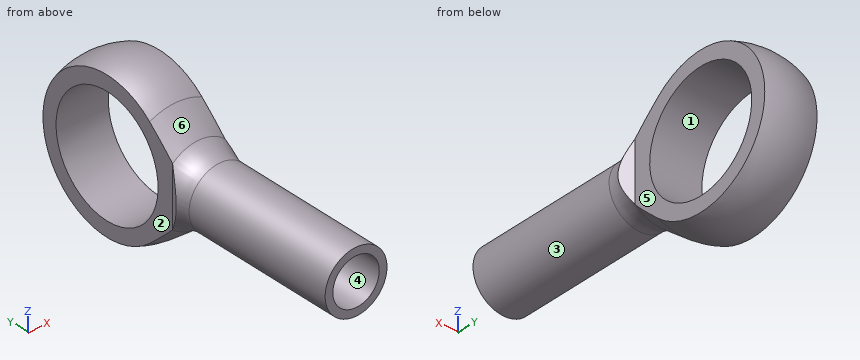
from build123d import *

# Parameters (mm, degrees)
CUT_EXTRUDE4_DEPTH      = 46.034307992
CUT_EXTRUDE4_DEPTH_BACK = 46.034307992
SKETCH3_R               = 7.5
CUT_EXTRUDE5_DEPTH      = 24
SKETCH5_R               = 3
CUT_EXTRUDE6_DEPTH      = 12.7


with BuildPart() as part:
    # Sketch1 → Revolve2 (revolve)
    with BuildSketch(Plane.XY, mode=Mode.PRIVATE) as revolve2_sk:
        with BuildLine():
            Line((0, 0), (0, 42.756156239))
            ThreePointArc((0, 42.756156239), (-9.01476789, 37.08443071), (-7.803677944, 26.502948219))
            Line((-7.803677944, 26.502948219), (-5.098161028, 23.12660401))
            ThreePointArc((-5.098161028, 23.12660401), (-4.282522133, 21.656925638), (-4, 20))
            Line((-4, 20), (-4, 0))
            Line((-4, 0), (0, 0))
        make_face()
    revolve(revolve2_sk.sketch.rotate(Axis((0, 0, 0), (0, 1, 0)), 270), axis=Axis((0, 0, 0), (0, 1, 0)))

    # Sketch2 → Cut-Extrude4 (cut, two sides: drawn at the far end of the back side and taken through both)
    with BuildSketch(Plane.XY.offset(-CUT_EXTRUDE4_DEPTH_BACK)):
        Polygon((-3.375, 42.756156239), (-20, 42.756156239), (-20, -5.668740666), (-3.375, 23.12660401), align=None)
        Polygon((20, 42.756156239), (3.375, 42.756156239), (3.375, 23.12660401), (20, -5.668740666), align=None)
    extrude(amount=CUT_EXTRUDE4_DEPTH + CUT_EXTRUDE4_DEPTH_BACK, mode=Mode.SUBTRACT)

    # Sketch3 → Cut-Extrude5 (cut)
    with BuildSketch(Plane(origin=(3.375, 0, 0), x_dir=(0, 0, -1), z_dir=(1, 0, 0))):
        with Locations((0, 32.756156239)):
            Circle(SKETCH3_R)
    extrude(amount=-CUT_EXTRUDE5_DEPTH, mode=Mode.SUBTRACT)

    # Sketch5 → Cut-Extrude6 (cut)
    with BuildSketch(Plane.XZ):
        with Locations(Location((0, 0, 0), (0, 0, 270))):
            Circle(SKETCH5_R)
    extrude(amount=-CUT_EXTRUDE6_DEPTH, mode=Mode.SUBTRACT)


solid = part.part
Design review of the part built by this model. Coordinates are the model's own, in mm. Face numbers are marked on the shaded views. A direction names the side the tool comes from. Coordinates: 2 decimals unless noted, no trailing zeros. Write each loop counter-clockwise with the first axis right and the second up, starting at its lowest first coordinate (ties: lowest second). Pieces come first, ordered by that corner, then holes. Notation, with made-up numbers: (-12.75, -30) - (-2.75, -30) arc R20 ccw to (-2.75, -3) - close; hole circle Ø11 at (-26, -19.5). An arc over 180 degrees is marked (long way). One line per item, written item: value.
1) Add section C-C (x = 0). State the section outline as (y, z) points.
Answer sheet:
outline: (0, -4) - (20, -4) arc R5 cw to (23.13, -5.1) - (26.5, -7.8) arc R10 ccw (long way) to (26.5, 7.8) - (23.13, 5.1) arc R5 cw to (20, 4) - (0, 4) - (0, 3) - (12.7, 3) - (12.7, -3) - (0, -3) - close; hole circle Ø15 at (32.76, 0)
2) Add section D-D (y = 8.5). State the section outline as (x, z) points.
Answer sheet:
outline: circle Ø8 at (0, 0); hole circle Ø6 at (0, 0)
3) Mouldability with a two-part tool opening along Z and no side actions: class the marked faces 1, 2, 3 and 4 as +Z half, -Z half, draft (parallel to the pull), parting line (faces both ways), or undercut.
Answer sheet:
face 1: undercut
face 2: draft
face 3: parting line
face 4: undercut
4) To check wall thickness, follow probe 1 along X at (y, z) = (9, 0); probe 2 along Y at (x, z) = (0, 0); probe 3 along X at (y, z) = (41, 3.25) (3 decimals). State the ranges of each line that lie inside material, in increasing order.
Answer sheet:
probe 1: x = -4 to -3, 3 to 4
probe 2: y = 12.7 to 25.26, 40.26 to 42.76
probe 3: x = -3.375 to 3.375
5) Add section A-A (z = 0). State the section outline as (x, y) points (1 decimal), plus the area to 3 significant figures.
Answer sheet:
outline: (-4.3, 21.6) arc R5 cw to (-4, 20) - (-4, 0) - (-3, 0) - (-3, 12.7) - (3, 12.7) - (3, 0) - (4, 0) - (4, 20) arc R5 cw to (4.3, 21.6) - (3.4, 23.1) - (3.4, 25.3) - (-3.4, 25.3) - (-3.4, 23.1) - close; (-3.4, 40.3) - (3.4, 40.3) - (3.4, 42.2) arc R10 ccw to (-3.4, 42.2) - close
area: 138 mm2
6) For the marked faces 5 and 6, list the 3-axis set-ups (+Z, -Z, +X, -X, +Y, -Y) from which the entire face can be reached by the end or side of a thin tool; tool diameter is ignored.
Answer sheet:
face 5: +Z, -Z, +X, +Y
face 6: +Z, -Y
7) Insertion check: pin 1 (1 mm diameter, centred on x = 3, y = 13, fed in from +Z); pin 2 (1 mm diameter, centred on y = 11, z = -1, fed in from -X); pin 3 (2 mm diameter, centred on y = 24.5, z = -5, fed in from +X) (3 decimals). Each pin has a flat end and moves straight along its axis. Give the tip position at first contact, or say it passes through.
Answer sheet:
pin 1: stops at z = 3.12
pin 2: stops at x = -3.97
pin 3: stops at x = 3.375
8) Add section B-B (y = 29.5). State the section outline as (x, z) points (3 decimals), plus the area to 3 significant figures.
Answer sheet:
outline: (-3.375, -8.832) arc R9.455 ccw to (3.375, -8.832) - (3.375, -6.756) - (-3.375, -6.756) - close; (-3.375, 6.756) - (3.375, 6.756) - (3.375, 8.832) arc R9.455 ccw to (-3.375, 8.832) - close
area: 33.7 mm2
